The drawing under review shows one solid part. Ordinate dimensions are in mm from its lowest x, y, z. Coordinates: 2 decimals unless noted, no trailing zeros. Loops run counter-clockwise (first coordinate to the right, second up) from the corner with the lowest first, then second, coordinate; pieces in that order, holes last. Notation, with made-up numbers: M 37,48 L 85,48 A5 ccw 85,55 Z; hole C 21,15 d9. An arc over 180 degrees is marked long. Answer as a JSON object with one key per item and string values. Group by question number.
1. Consider section C-C (x = 25.5). State the section outline as (y, z) points, then the cut area to 3 significant figures.
2. Consider section A-A (y = 5). State the section outline as (x, z) points, then the cut area to 3 significant figures.
3. Insertion check: pin 1 (5 mm diameter, centred on x = 24.5, y = 12, fed in from +Z); pin 2 (0.5 mm diameter, centred on x = 13.5, z = 0.5, fed in from +Y). Each pin has a flat end and moves straight along its axis. Give the tip position at first contact, or say it passes through.
4. To check wall thickness, follow probe 1 along Z at (x, y) = (8, 29); probe 2 along Y at (x, z) = (36.5, 1.5); probe 3 along Y at (x, z) = (26, 5.25). State the ranges of each line that lie inside material, in increasing order.
5. Consider section B-B (x = 12.5). State the section outline as (y, z) points, then the cut area to 3 significant figures.
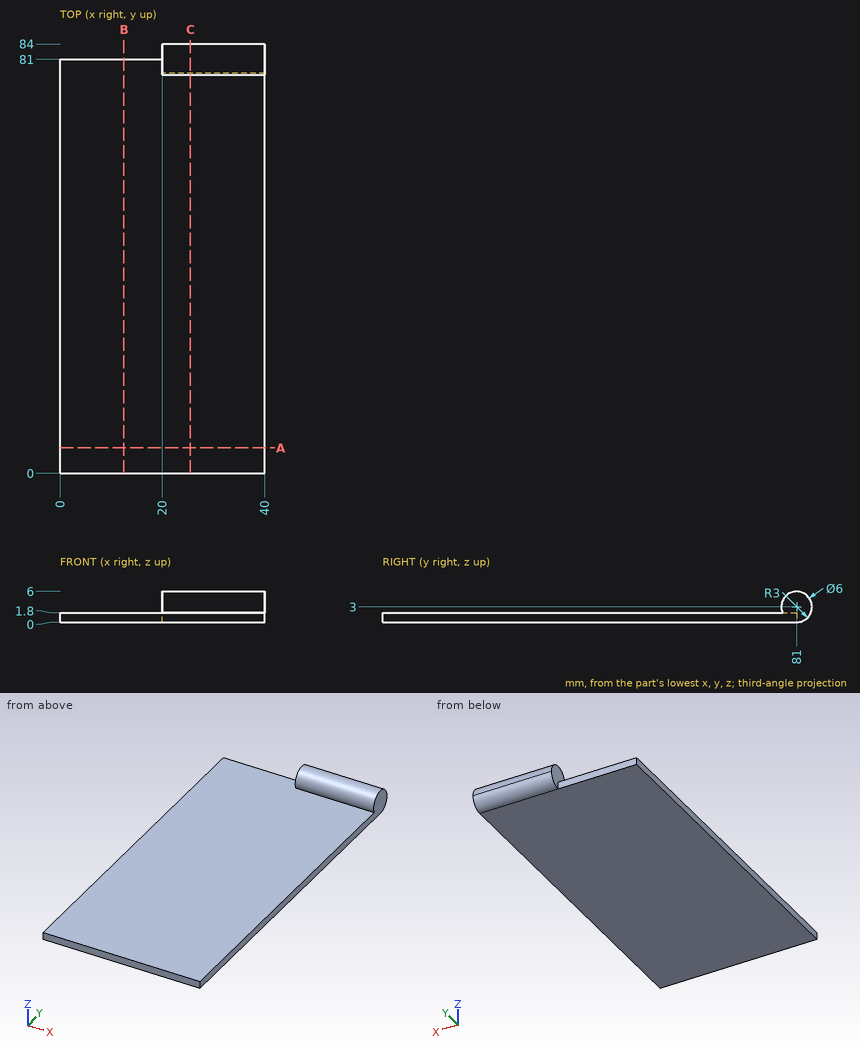
Findings below:
{
 "1": {"outline": "M 0,0 L 81,0 A3 ccw long 78.25,1.8 L 0,1.8 Z", "area": "171 mm^2"},
 "2": {"outline": "M 0,0 L 40,0 L 40,1.8 L 0,1.8 Z", "area": "72.0 mm^2"},
 "3": {"pin 1": "stops at z = 1.8", "pin 2": "stops at y = 81"},
 "4": {"probe 1": "z = 0 to 1.8", "probe 2": "y = 0 to 83.6", "probe 3": "y = 79.02 to 82.98"},
 "5": {"outline": "M 0,0 L 81,0 L 81,1.8 L 0,1.8 Z", "area": "146 mm^2"}
}
